The drawing under review shows one solid part. Ordinate dimensions are in mm from its lowest x, y, z. A direction names the side the tool comes from. Give positions to 0.01 mm unless a question says otherwise; leave off trailing zeros. Order: outer loops, then holes, each group sorted by start corner. A loop starts at its lowest first (then second) coordinate and runs counter-clockwise, first axis right, second up. Notation, with made-up numbers: (-9, 74.5) - (23, 74.5) arc R23 ccw to (23, 105.5) - close; hole circle Ø6 at (87.25, -22). An arc over 180 degrees is marked (long way). Answer as a JSON object with one key per item and string values. Group by question number.
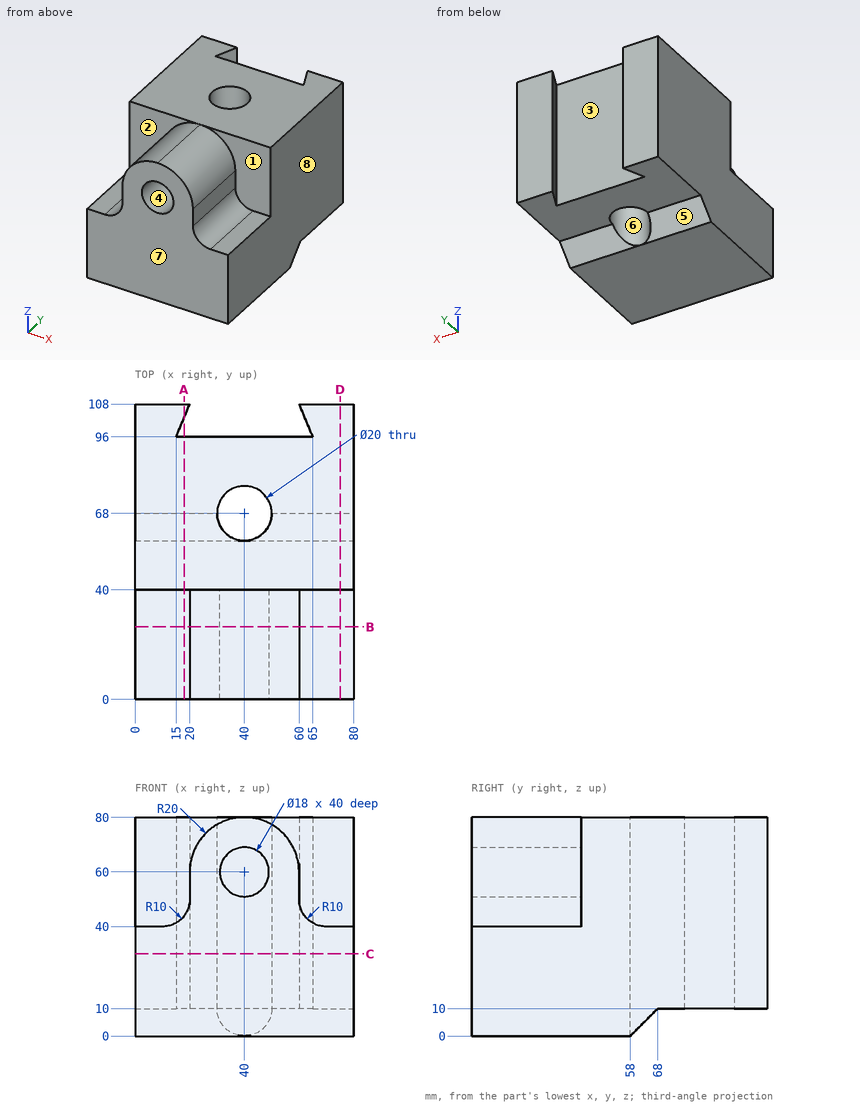
1) Consider section D-D (x = 75). Give the boundary of the cut face in (y, z).
2) For the marked faces 1, 2, 3 and 4, list the 3-axis set-ups (+Z, -Z, +X, -X, +Y, -Y) from which the entire face can be reached by the end or side of a thin tool; tool diameter is ignored.
3) Consider section B-B (y = 26.5). Give the boundary of the cut face in (x, z).
4) Consider section C-C (z = 30). Give the boundary of the cut face in (x, y), plus the area to 3 significant figures.
5) For line 1 (Z direction, x = 40, y = 31); line 2 (Y direction, x = 40, z = 35); line 3 (Z direction, x = 6.5, y = 14), list the stretches that pass through material, from the lowest coordinate up.
6) Mouldability with a two-part tool opening along Y and no side actions: class the marked faces 5, 6, 7 and 8 as released by +Y, released by -Y, zero draft, split by the parting line, or undercut.
7) For pin 1 (4 mm diameter, centred on x = 28, z = 14, fed in from +Y); pin 2 (20 mm diameter, centred on x = 34.5, y = 98, fed in from -Z); pin 3 (3 mm diameter, centred on y = 18.5, z = 53, fed in from +X), all flat-tipped, find the tip position at first contact; note any pin that passes through.
8) Consider section A-A (x = 18). Give the boundary of the cut face in (y, z), plus the area to 3 significant figures.
Result set:
{
 "1": {"outline": "(0, 0) - (58, 0) - (68, 10) - (108, 10) - (108, 80) - (40, 80) - (40, 40) - (0, 40) - close"},
 "2": {"face 1": "+Z, +X, -Y", "face 2": "+Z, -X, -Y", "face 3": "+Z, -Z", "face 4": "-Y"},
 "3": {"outline": "(0, 0) - (80, 0) - (80, 40) - (70, 40) arc R10 cw to (60, 50) - (60, 60) arc R20 ccw to (20, 60) - (20, 50) arc R10 cw to (10, 40) - (0, 40) - close; hole circle Ø18 at (40, 60)"},
 "4": {"outline": "(0, 0) - (80, 0) - (80, 108) - (60, 108) - (65, 96) - (15, 96) - (20, 108) - (0, 108) - close; hole circle Ø20 at (40, 68)", "area": "7,790 mm2"},
 "5": {"line 1": "z = 0 to 51, 69 to 80", "line 2": "y = 0 to 58, 78 to 96", "line 3": "z = 0 to 40"},
 "6": {"face 5": "released by +Y", "face 6": "undercut", "face 7": "released by -Y", "face 8": "zero draft"},
 "7": {"pin 1": "stops at y = 96", "pin 2": "stops at z = 10", "pin 3": "stops at x = 60"},
 "8": {"outline": "(0, 0) - (58, 0) - (68, 10) - (96, 10) - (96, 80) - (40, 80) - (40, 44) - (0, 44) - close; (103.2, 10) - (108, 10) - (108, 80) - (103.2, 80) - close", "area": "6,250 mm2"}
}
